Geometry check sheet. Reference: the model listing, model coordinates, mm. A direction names the side the tool comes from. Give positions to 0.01 mm unless a question says otherwise; leave off trailing zeros. Order: outer loops, then holes, each group sorted by start corner. A loop starts at its lowest first (then second) coordinate and runs counter-clockwise, first axis right, second up.
from build123d import *

# Parameters (mm, degrees)
BOSS_EXTRUDE1_DEPTH   = 4.7625
M8_CLEARANCE_HOLE1_D  = 9
M4X0_7_TAPPED_HOLE2_D = 3.3
CHAMFER1_SIZE         = 1


with BuildPart() as part:
    # Sketch1 → Boss-Extrude1 (new, symmetric)
    with BuildSketch(Plane(origin=(0, 0, 0), x_dir=(1, 0, 0), z_dir=(0, 1, 0))):
        with BuildLine():
            Line((20, 0), (20, 28))
            Line((20, 28), (80, 28))
            Line((80, 28), (80, -72))
            Line((80, -72), (-80, -72))
            Line((-80, -72), (-80, 28))
            Line((-80, 28), (-20, 28))
            Line((-20, 28), (-20, 0))
            ThreePointArc((-20, 0), (0, -20), (20, 0))
        make_face()
    extrude(amount=BOSS_EXTRUDE1_DEPTH, both=True)

    # M8 Clearance Hole1 (through all)
    with Locations(Plane(origin=(0, 4.7625, 0), x_dir=(1, 0, 0), z_dir=(0, 1, 0))):
        with Locations((-40, -57), (0, -57), (40, -57)):
            Hole(M8_CLEARANCE_HOLE1_D / 2)

    # M4x0.7 Tapped Hole2 (through all)
    with Locations(Plane(origin=(0, 4.7625, 0), x_dir=(1, 0, 0), z_dir=(0, 1, 0))):
        with Locations((-23.573172318, -23.573172318), (-23.573172318, 23.573172318), (23.573172318, 23.573172318), (23.573172318, -23.573172318)):
            Hole(M4X0_7_TAPPED_HOLE2_D / 2)

    # Chamfer1
    chamfer1_edges = [part.edges().sort_by_distance(p)[0] for p in [
        (80, 0, -28),
        (80, 0, 72),
        (-80, 0, 72),
        (-80, 0, -28),
    ]]
    chamfer(chamfer1_edges, length=CHAMFER1_SIZE)


solid = part.part
Item 1: Sectioned sample at B-B (z = 57). Enter the section's corners in (x, y), and give its area (3 significant figures).
Reported:
outline: (-80, -4.76) - (-44.5, -4.76) - (-44.5, 4.76) - (-80, 4.76) - close; (-35.5, -4.76) - (-4.5, -4.76) - (-4.5, 4.76) - (-35.5, 4.76) - close; (4.5, -4.76) - (35.5, -4.76) - (35.5, 4.76) - (4.5, 4.76) - close; (44.5, -4.76) - (80, -4.76) - (80, 4.76) - (44.5, 4.76) - close
area: 1,270 mm2
Item 2: Sectioned sample at C-C (z = -12). Enter the section's corners in (x, y).
Reported:
outline: (-80, -4.76) - (-20, -4.76) - (-20, 4.76) - (-80, 4.76) - close; (20, -4.76) - (80, -4.76) - (80, 4.76) - (20, 4.76) - close
Item 3: Set-up check for faces 1 (the flat face through (49, 0, -28)), 2 (the flat face through (20, 0, -14)): record each of +Z, -Z, +X, -X, +Y, -Y from which the full face is reachable in a straight line by a thin tool's end or side.
Reported:
face 1: -Z, +X, -X, +Y, -Y
face 2: -Z, +Y, -Y
Item 4: Sectioned sample at D-D (y = 3). Enter the section's corners in (x, z), and give its area (3 significant figures).
Reported:
outline: (-80, -27) - (-79, -28) - (-20, -28) - (-20, 0) arc R20 cw to (20, 0) - (20, -28) - (79, -28) - (80, -27) - (80, 71) - (79, 72) - (-79, 72) - (-80, 71) - close; hole circle Ø9 at (-40, 57); hole circle Ø3.3 at (-23.57, -23.57); hole circle Ø3.3 at (-23.57, 23.57); hole circle Ø9 at (0, 57); hole circle Ø3.3 at (23.57, -23.57); hole circle Ø3.3 at (23.57, 23.57); hole circle Ø9 at (40, 57)
area: 14,000 mm2
Item 5: Scan lines: L1, parallel to X at y = 3.5, z = -1; L2, parallel to X at y = 3, z = 57; L3, parallel to Z at x = -0.5, y = 3.25. Record each from-to range of solid material in increasing order.
Reported:
L1: x = -80 to -20, 20 to 80
L2: x = -80 to -44.5, -35.5 to -4.5, 4.5 to 35.5, 44.5 to 80
L3: z = 19.99 to 52.53, 61.47 to 72
Item 6: Sectioned sample at A-A (x = 0). Enter the section's corners in (y, z).
Reported:
outline: (-4.76, 20) - (4.76, 20) - (4.76, 52.5) - (-4.76, 52.5) - close; (-4.76, 61.5) - (4.76, 61.5) - (4.76, 72) - (-4.76, 72) - close
